from build123d import *

# Parameters (mm, degrees)
F0_R     = 10
F1_DEPTH = 25
F2_DEPTH = 50
F3_SIZE  = 1
F4_SIZE  = 1


with BuildPart() as f1:
    # F0 (on Front) → F1 (new body)
    with BuildSketch(Plane.XZ):
        with BuildLine():
            ThreePointArc((2.777778, -24.8452), (18.6339, -16.666667), (25, 0))
            ThreePointArc((25, 0), (18.6339, 16.666667), (2.777778, 24.8452))
            ThreePointArc((2.777778, 24.8452), (-25, 0), (2.777778, -24.8452))
        make_face()
        Circle(F0_R, mode=Mode.SUBTRACT)
        with BuildLine():
            ThreePointArc((2.777778, 24.8452), (18.6339, 16.666667), (25, 0))
            ThreePointArc((25, 0), (18.6339, -16.666667), (2.777778, -24.8452))
            Line((2.777778, -24.8452), (91.666667, -14.90712))
            ThreePointArc((91.666667, -14.90712), (75, 0), (91.666667, 14.90712))
            Line((91.666667, 14.90712), (2.777778, 24.8452))
        make_face()
        with BuildLine():
            ThreePointArc((105, 0), (101.18034, 10), (91.666667, 14.90712))
            ThreePointArc((91.666667, 14.90712), (75, 0), (91.666667, -14.90712))
            ThreePointArc((91.666667, -14.90712), (101.18034, -10), (105, 0))
        make_face()
        with Locations((90, 0)):
            Circle(F0_R, mode=Mode.SUBTRACT)
    extrude(amount=F1_DEPTH)

    # F0 (on Front) → F2 (join)
    with BuildSketch(Plane.XZ):
        with BuildLine():
            ThreePointArc((2.777778, -24.8452), (18.6339, -16.666667), (25, 0))
            ThreePointArc((25, 0), (18.6339, 16.666667), (2.777778, 24.8452))
            ThreePointArc((2.777778, 24.8452), (-25, 0), (2.777778, -24.8452))
        make_face()
        Circle(F0_R, mode=Mode.SUBTRACT)
    extrude(amount=F2_DEPTH)

    # F3
    f3_edges = [f1.edges().sort_by_distance(p)[0] for p in [
        (-2.777778, -50, 24.8452),
    ]]
    chamfer(f3_edges, length=F3_SIZE)

    # F4
    f4_edges = [f1.edges().sort_by_distance(p)[0] for p in [
        (80, -25, 0),
        (-10, -50, 0),
    ]]
    chamfer(f4_edges, length=F4_SIZE)


solid = f1.part
Model file for the job. Use its own axes, mm. Give positions to 0.01 mm unless a question says otherwise; leave off trailing zeros. Write each loop counter-clockwise with the first axis right and the second up, starting at its lowest first coordinate (ties: lowest second). Pieces come first, ordered by that corner, then holes. Notation, with made-up numbers: (-3.5, 20.5) -> (33.5, 20.5) arc R16 cw to (33.5, 30.5) -> close; hole circle Ø2 at (32, 81.5). An arc over 180 degrees is marked (long way). Write item = value, one per line.
(1) Probe line 1 along Z through (x, y) = (0, -9); line 2 along X through (y, z) = (-20, -8.5); line 3 along Y through (x, z) = (47, 0). List the from-to ranges inside material, lowest first.
Determined:
line_1 = -25 to -10, 10 to 25
line_2 = -23.51 to -5.27, 5.27 to 84.73, 95.27 to 102.36
line_3 = -25 to 0
(2) Slice it at C-C, the plane x = 90. Give the cut face in (y, z), then the cut area to 3 significant figures.
Determined:
outline = (-25, -15.09) -> (0, -15.09) -> (0, -10) -> (-24, -10) -> (-25, -11) -> close; (-25, 11) -> (-24, 10) -> (0, 10) -> (0, 15.09) -> (-25, 15.09) -> close
area = 254 mm2
(3) Slice it at A-A, the plane y = -14. Give the cut face in (x, z), then the cut area to 3 significant figures.
Determined:
outline = (2.78, -24.85) -> (91.67, -14.91) arc R15 ccw to (91.67, 14.91) -> (2.78, 24.85) arc R25 ccw (long way) to start; hole circle Ø20 at (0, 0); hole circle Ø20 at (90, 0)
area = 4,330 mm2
(4) Flat gauge pins, fed straight in: P1, Ø3, axis at y = -18, z = -5.5, coming from the -X side; P2, Ø10, axis at y = -32.5, z = 18, coming from the -X side; P3, Ø3, axis at x = 27, z = -10.5, coming from the +Y side; P4, Ø12, axis at x = 90, z = 0, coming from the +Y side. Where does each tip first touch, or does it go through?
Determined:
P1 = -24.68
P2 = -21.35
P3 = 0
P4 = through
(5) Slice it at D-D, the plane z = 7. Give the number of separate pieces and of enclosed holes in the cut face, then the cut area to 3 significant figures.
Determined:
separate_pieces = 3
enclosed_holes = 0
area = 3,310 mm2
(6) Slice it at B-B, the plane y = -30. Give the cut face in (x, z).
Determined:
outline = circle Ø50 at (0, 0); hole circle Ø20 at (0, 0)
(7) Mould opens along Z. For faces 1 (the face through (46.6, -12.325, -19.946)), 2 (the face through (80, -12, 0)), 3 (the face through (10, -50, -5)) say: released by +Z, released by -Z, zero draft, split by the parting line, or undercut.
Determined:
face_1 = released by -Z
face_2 = undercut
face_3 = zero draft
